Input: part model. Units: mm. Frame: model coordinates. Face numbers are marked on the shaded views. A direction names the side the tool comes from. Give positions to 0.01 mm unless a question says otherwise; leave off trailing zeros. Order: outer loops, then holes, each group sorted by start corner. A loop starts at its lowest first (then second) coordinate and runs counter-clockwise, first axis right, second up. Notation, with made-up numbers: (-27.75, 61.5) - (24.25, 61.5) arc R31 cw to (24.25, 87.5) - close; hole circle Ø4 at (11, 78.5). An arc over 180 degrees is marked (long way). Answer in a Markdown table with one row per item. Add a question column.
1. Section query B-B on x = 0. Return loops of the section in (y, z) (3 decimals).
2. Section query C-C on z = 15. Return loops of the section in (x, y) (3 decimals).
3. Ray query, line 1 (Y direction, x = 0, z = 9) (3 decimals); line 2 (Y direction, x = 0, z = 57); line 3 (Y direction, x = 11.5, z = 16.5). Return the intervals inside material, ascending. Write a range as [from, to].
4. Access query for the marked faces 1, 2 and 3. Directions: +Z, -Z, +X, -X, +Y, -Y. A direction counts if a zero-diameter tool reaches every point of the face in a straight line with its end or side. Return the directions, or none.
5. Mould query, pull axis Y, two halves, no side actions, for the marked faces 4, 5 and 6. Classes: released by +Y, released by -Y, zero draft, split by the parting line, or undercut.
6. Contact query for flat-ended pins moving along their axis: pin 1 (3 mm diameter, centred on x = 13, y = -21, fed in from +Z); pin 2 (9.5 mm diameter, centred on x = 0.5, z = 32.5, fed in from -Y); pin 3 (3.5 mm diameter, centred on x = -1.5, z = 32.5, fed in from +Y); pin 4 (9 mm diameter, centred on x = 0, y = 0, fed in from -Z). Output: stop coordinate, or through.
7. Section query A-A on z = 59. Return loops of the section in (x, y).
```python
from build123d import *

# Parameters (mm, degrees)
F0_R     = 37.325
F1_DEPTH = 20
F2_R     = 33.325
F2_R_2   = 19.325
F3_DEPTH = 15
F4_W     = 15
F4_H     = 15
F5_DEPTH = 45
F6_SIZE2 = 3
F6_SIZE  = 3
F7_R     = 4
F8_DEPTH = 10


with BuildPart() as f1:
    # F0 (on Top) → F1 (new body)
    with BuildSketch(Plane.XY):
        Circle(F0_R)
    extrude(amount=F1_DEPTH)

    # F2 (on face) → F3 (cut)
    with BuildSketch(Plane.XY.offset(20)):
        Circle(F2_R)
        Circle(F2_R_2, mode=Mode.SUBTRACT)
    extrude(amount=-F3_DEPTH, mode=Mode.SUBTRACT)

    # F4 (on face) → F5 (join)
    with BuildSketch(Plane.XY.offset(20)):
        Rectangle(F4_W, F4_H)
    extrude(amount=F5_DEPTH)

    # F6
    f6_edges = [f1.edges().sort_by_distance(p)[0] for p in [
        (7.5, 7.5, 42.5),
        (7.5, -7.5, 42.5),
    ]]
    chamfer(f6_edges, length=F6_SIZE, length2=F6_SIZE2)

    # F7 (on face) → F8 (cut)
    with BuildSketch(Plane.XY.offset(65)):
        Circle(F7_R)
    extrude(amount=-F8_DEPTH, mode=Mode.SUBTRACT)


solid = f1.part
```
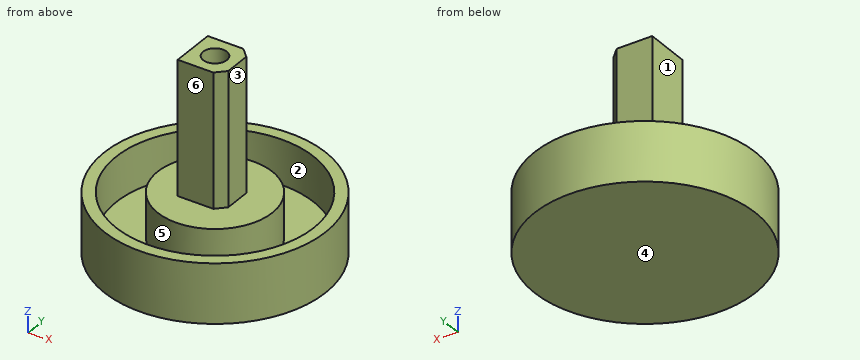
Answer:
| question | item | result |
|---|---|---|
| 1 | outline | (-37.325, 0) - (37.325, 0) - (37.325, 20) - (33.325, 20) - (33.325, 5) - (19.325, 5) - (19.325, 20) - (7.5, 20) - (7.5, 65) - (4, 65) - (4, 55) - (-4, 55) - (-4, 65) - (-7.5, 65) - (-7.5, 20) - (-19.325, 20) - (-19.325, 5) - (-33.325, 5) - (-33.325, 20) - (-37.325, 20) - close |
| 2 | outline | circle Ø74.65 at (0, 0); circle Ø38.65 at (0, 0); hole circle Ø66.65 at (0, 0) |
| 3 | line 1 | y = [-37.325, -33.325], [-19.325, 19.325], [33.325, 37.325] |
| 3 | line 2 | y = [-7.5, -4], [4, 7.5] |
| 3 | line 3 | y = [-35.51, -31.28], [-15.53, 15.53], [31.28, 35.51] |
| 4 | face 1 | +Z, -X, +Y, -Y |
| 4 | face 2 | +Z |
| 4 | face 3 | +Z, +X, +Y, -Y |
| 5 | face 4 | zero draft |
| 5 | face 5 | undercut |
| 5 | face 6 | released by -Y |
| 6 | pin 1 | stops at z = 5 |
| 6 | pin 2 | stops at y = -7.5 |
| 6 | pin 3 | stops at y = 7.5 |
| 6 | pin 4 | stops at z = 0 |
| 7 | outline | (-7.5, -7.5) - (4.5, -7.5) - (7.5, -4.5) - (7.5, 4.5) - (4.5, 7.5) - (-7.5, 7.5) - close; hole circle Ø8 at (0, 0) |
